Can you work these out from the model? Positions are in its coordinate system, mm. Coordinates: 2 decimals unless noted, no trailing zeros. Loops run counter-clockwise (first coordinate to the right, second up) from the corner with the lowest first, then second, coordinate; pieces in that order, holes last. Notation, with made-up numbers: M 69.5,-32 L 76.5,-32 A16 cw 76.5,-8 Z; hole C -7,13 d6. An arc over 180 degrees is marked long. Return JSON: item names as keys, results as strings. Group by question number.
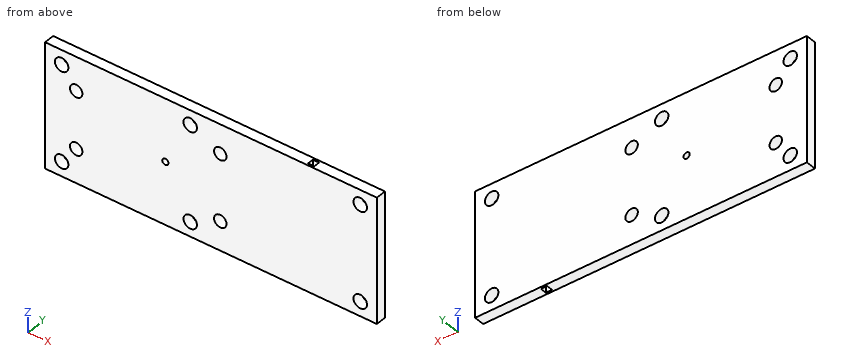
```python
from build123d import *

# Parameters (mm, degrees)
SKETCH1_W           = 160
SKETCH1_H           = 60
SKETCH1_R           = 3.25
SKETCH1_R_2         = 3
SKETCH1_R_3         = 1.5
BOSS_EXTRUDE1_DEPTH = 5
SKETCH2_W           = 3
SKETCH2_H           = 3
CUT_1EXTRUDE1_DEPTH = 65


with BuildPart() as part:
    # Sketch1 → Boss-Extrude1 (new body)
    with BuildSketch(Plane(origin=(0, 0, 0), x_dir=(1, 0, 0), z_dir=(0, 1, 0))):
        Rectangle(SKETCH1_W, SKETCH1_H)
        with Locations(Location((-72, 23, 0), (0, 0, 270))):
            Circle(SKETCH1_R, mode=Mode.SUBTRACT)
        with Locations(Location((-72, -23, 0), (0, 0, 270))):
            Circle(SKETCH1_R, mode=Mode.SUBTRACT)
        with Locations(Location((72, 23, 0), (0, 0, 270))):
            Circle(SKETCH1_R, mode=Mode.SUBTRACT)
        with Locations(Location((72, -23, 0), (0, 0, 270))):
            Circle(SKETCH1_R, mode=Mode.SUBTRACT)
        with Locations(Location((-10, 23, 0), (0, 0, 270))):
            Circle(SKETCH1_R, mode=Mode.SUBTRACT)
        with Locations(Location((-10, -23, 0), (0, 0, 270))):
            Circle(SKETCH1_R, mode=Mode.SUBTRACT)
        with Locations(Location((4.5, 16, 0), (0, 0, 270))):
            Circle(SKETCH1_R_2, mode=Mode.SUBTRACT)
        with Locations(Location((4.5, -16, 0), (0, 0, 270))):
            Circle(SKETCH1_R_2, mode=Mode.SUBTRACT)
        with Locations(Location((-65, 13.75, 0), (0, 0, 270))):
            Circle(SKETCH1_R_2, mode=Mode.SUBTRACT)
        with Locations(Location((-65, -13.75, 0), (0, 0, 270))):
            Circle(SKETCH1_R_2, mode=Mode.SUBTRACT)
        with Locations(Location((-22, 0, 0), (0, 0, 270))):
            Circle(SKETCH1_R_3, mode=Mode.SUBTRACT)
    extrude(amount=BOSS_EXTRUDE1_DEPTH)

    # Sketch2 → Cut-1Extrude1 (cut)
    with BuildSketch(Plane.XY.offset(30)):
        with Locations((47.530607127, 2.5)):
            Rectangle(SKETCH2_W, SKETCH2_H)
    extrude(amount=-CUT_1EXTRUDE1_DEPTH, mode=Mode.SUBTRACT)


solid = part.part
```
1) If I drill on line 1 (X direction, y = 3.65, z = -23); line 2 (X direction, y = 1.35, z = -8); line 3 (Y direction, x = 46.5, z = -6), over which ranges is the centre line in solid material (lowest first)? Write a range as from..to.
2) Suppose I cut it at B-B, the plane x = -22. List the corners of the cut face in (y, z) for me.
3) Suppose I cut it at A-A, the plane z = 0. List the corners of the cut face in (x, y) for me, then the cut area to 3 significant figures.
4) For pin 1 (6 mm diameter, centred on x = -72, z = 23, fed in from +Y); pin 2 (7 mm diameter, centred on x = -65, z = 13.75, fed in from -Y), each with a flat end and sliding along its axis, tell me the tip position at first contact or that it passes through.
5) Suppose I cut it at D-D, the plane z = -23. List the corners of the cut face in (x, y) for me, then the cut area to 4 significant figures.
6) Suppose I cut it at C-C, the plane x = 4.5. List the corners of the cut face in (y, z) for me, then the cut area to 3 significant figures.
Returned:
{
 "1": {"line 1": "x = -80..-75.25, -68.75..-13.25, -6.75..46.03, 49.03..68.75, 75.25..80", "line 2": "x = -80..46.03, 49.03..80", "line 3": "y = 0..1, 4..5"},
 "2": {"outline": "M 0,-30 L 5,-30 L 5,-1.5 L 0,-1.5 Z; M 0,1.5 L 5,1.5 L 5,30 L 0,30 Z"},
 "3": {"outline": "M -80,0 L -23.5,0 L -23.5,5 L -80,5 Z; M -20.5,0 L 80,0 L 80,5 L -20.5,5 Z; hole M 46.03,1 L 49.03,1 L 49.03,4 L 46.03,4 Z", "area": "776 mm²"},
 "4": {"pin 1": "passes through", "pin 2": "stops at y = 0"},
 "5": {"outline": "M -80,0 L -75.25,0 L -75.25,5 L -80,5 Z; M -68.75,0 L -13.25,0 L -13.25,5 L -68.75,5 Z; M -6.75,0 L 68.75,0 L 68.75,5 L -6.75,5 Z; M 75.25,0 L 80,0 L 80,5 L 75.25,5 Z; hole M 46.03,1 L 49.03,1 L 49.03,4 L 46.03,4 Z", "area": "693.5 mm²"},
 "6": {"outline": "M 0,-30 L 5,-30 L 5,-19 L 0,-19 Z; M 0,-13 L 5,-13 L 5,13 L 0,13 Z; M 0,19 L 5,19 L 5,30 L 0,30 Z", "area": "240 mm²"}
}
